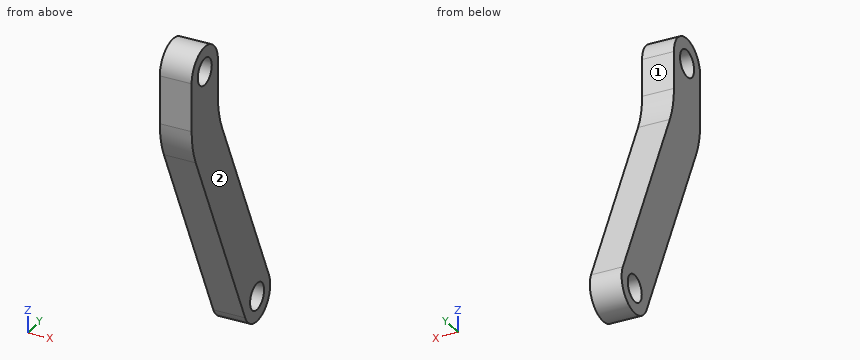
from build123d import *

# Parameters (mm, degrees)
SKETCH1_R           = 1.6
BOSS_EXTRUDE1_DEPTH = 1.9


with BuildPart() as part:
    # Sketch1 → Boss-Extrude1 (new, symmetric)
    with BuildSketch(Plane(origin=(0, 0, 0), x_dir=(0, 0, -1), z_dir=(1, 0, 0))):
        with BuildLine():
            Line((0, -3), (5.789792528, -3))
            ThreePointArc((5.789792528, -3), (7.947916139, -2.764348543), (10.004326756, -2.068500496))
            Line((10.004326756, -2.068500496), (34.314360268, 9.229449851))
            ThreePointArc((34.314360268, 9.229449851), (35.770550149, 13.214360268), (31.785639732, 14.670550149))
            Line((31.785639732, 14.670550149), (8.678202272, 3.931499504))
            ThreePointArc((8.678202272, 3.931499504), (6.621791656, 3.235651457), (4.463668044, 3))
            Line((4.463668044, 3), (0, 3))
            ThreePointArc((0, 3), (-3, 0), (0, -3))
        make_face()
        with Locations(Location((0, 0, 0), (0, 0, 180))):
            Circle(SKETCH1_R, mode=Mode.SUBTRACT)
        with Locations(Location((33.05, 11.95, 0), (0, 0, 180))):
            Circle(SKETCH1_R, mode=Mode.SUBTRACT)
    extrude(amount=BOSS_EXTRUDE1_DEPTH, both=True)


solid = part.part
Geometry check sheet. Reference: the model listing, model coordinates, mm. Face numbers are marked on the shaded views. A direction names the side the tool comes from. Give positions to 0.01 mm unless a question says otherwise; leave off trailing zeros. Loops run counter-clockwise (first coordinate to the right, second up) from the corner with the lowest first, then second, coordinate; pieces in that order, holes last. Notation, with made-up numbers: (13.5, 84) -> (57.5, 84) arc R8 cw to (57.5, 99) -> close; hole circle Ø4 at (2, -4). An arc over 180 degrees is marked (long way). Answer in a Markdown table with one row per item. Add a question column.
1) Cross-section at C-C on z = -33.05. Record the boundary of the cut face in (x, y), and give its area (3 significant figures).
2) Gauge pin test, flat ends, axial feed: P1, Ø5, axis at y = 11.95, z = -33.05, coming from the -X side; P2, Ø2, axis at x = 0.5, z = -24, coming from the -Y side; P3, Ø2, axis at x = 0.5, z = -30.5, coming from the -Y side; P4, Ø1.9, axis at x = 0, z = -3, coming from the +Y side. Record the tip position at first contact, or that the pin passes through.
3) Cross-section at A-A on x = 0.2. Record the boundary of the cut face in (y, z), and give its area (3 significant figures).
4) Cross-section at D-D on z = -27. Record the boundary of the cut face in (x, y).
5) Set-up check for the marked faces 1 and 2: record each of +Z, -Z, +X, -X, +Y, -Y from which the full face is reachable in a straight line by a thin tool's end or side.
6) Material ranges on probe 1 along Y at (x, z) = (-0.55, 0); probe 2 along Z at (x, y) = (-0.85, 1); probe 3 along Z at (x, y) = (0.35, -1), recorded low to high. Write a range as from..to.
7) Cross-section at B-B on y = 11.95. Record the boundary of the cut face in (x, z), and give its area (3 significant figures).
Outcome:
| question | item | result |
|---|---|---|
| 1 | outline | (-1.9, 8.64) -> (1.9, 8.64) -> (1.9, 10.35) -> (-1.9, 10.35) -> close; (-1.9, 13.55) -> (1.9, 13.55) -> (1.9, 14.95) -> (-1.9, 14.95) -> close |
| 1 | area | 11.8 mm^2 |
| 2 | P1 | stops at x = -1.9 |
| 2 | P2 | stops at y = 3.97 |
| 2 | P3 | stops at y = 6.99 |
| 2 | P4 | stops at y = 3 |
| 3 | outline | (-3, -5.79) arc R10 ccw to (-2.07, -10) -> (9.23, -34.31) arc R3 ccw to (14.67, -31.79) -> (3.93, -8.68) arc R10 cw to (3, -4.46) -> (3, 0) arc R3 ccw to (-3, 0) -> close; hole circle Ø3.2 at (0, 0); hole circle Ø3.2 at (11.95, -33.05) |
| 3 | area | 226 mm^2 |
| 4 | outline | (-1.9, 5.83) -> (1.9, 5.83) -> (1.9, 12.45) -> (-1.9, 12.45) -> close |
| 5 | face 1 | +Z, +X, -X, +Y |
| 5 | face 2 | +Z, -Z, +X, +Y, -Y |
| 6 | probe 1 | y = -3..-1.6, 1.6..3 |
| 6 | probe 2 | z = -16.61..-1.25, 1.25..2.83 |
| 6 | probe 3 | z = -12.3..-1.25, 1.25..2.83 |
| 7 | outline | (-1.9, -36.05) -> (1.9, -36.05) -> (1.9, -34.65) -> (-1.9, -34.65) -> close; (-1.9, -31.45) -> (1.9, -31.45) -> (1.9, -25.93) -> (-1.9, -25.93) -> close |
| 7 | area | 26.3 mm^2 |
